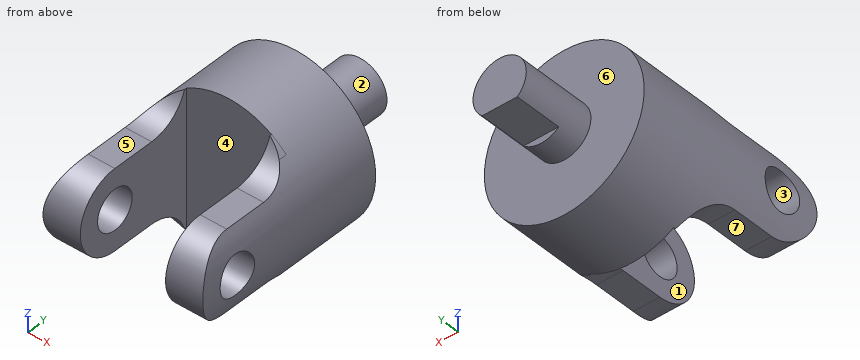
from build123d import *

# Parameters (mm, degrees)
IZIM2_R                          = 19.05
Y_KSEKLIK_EKSTR_ZYON2_DEPTH      = 18.42
Y_KSEKLIK_EKSTR_ZYON4_REACH      = 41.439
Y_KSEKLIK_EKSTR_ZYON4_END_RADIUS = 19.05
IZIM3_R                          = 4.765
RADYUS1_R                        = 9.53
IZIM5_R                          = 6.35
Y_KSEKLIK_EKSTR_ZYON5_DEPTH      = 17.81
IZIM6_W                          = 1.59
IZIM6_H                          = 11.43
KES_EKSTR_ZYON2_DEPTH            = 8.905


with BuildPart() as part:
    # Çizim2 → Yükseklik-Ekstrüzyon2 (new body)
    with BuildSketch(Plane(origin=(0, 0, 0), x_dir=(1, 0, 0), z_dir=(0, 1, 0))):
        with Locations(Location((0, 0, 0), (0, 0, 270))):
            Circle(IZIM2_R)
    extrude(amount=-Y_KSEKLIK_EKSTR_ZYON2_DEPTH)

    # Yükseklik-Ekstrüzyon4: up to this cylinder (the profile starts inside it)
    y_kseklik_ekstr_zyon4_end = Plane(origin=(0, -31.124737, 0), z_dir=(0, 1, 0)) * Cylinder(Y_KSEKLIK_EKSTR_ZYON4_END_RADIUS, 121.978, mode=Mode.PRIVATE)
    # Çizim3 → Yükseklik-Ekstrüzyon4 (add, up to the surface)
    with BuildSketch(Plane(origin=(10.16, 0, 0), x_dir=(0, 0, -1), z_dir=(1, 0, 0)), mode=Mode.PRIVATE) as y_kseklik_ekstr_zyon4_sk1:
        with BuildLine():
            Line((-9.53, -38.1), (-9.53, -18.42))
            Line((-9.53, -18.42), (9.53, -18.42))
            Line((9.53, -18.42), (9.53, -38.1))
            ThreePointArc((9.53, -38.1), (0, -47.63), (-9.53, -38.1))
        make_face()
        with Locations(Location((0, -38.1, 0), (0, 0, 180))):
            Circle(IZIM3_R, mode=Mode.SUBTRACT)
    y_kseklik_ekstr_zyon4_tool1 = extrude(y_kseklik_ekstr_zyon4_sk1.sketch, amount=Y_KSEKLIK_EKSTR_ZYON4_REACH, mode=Mode.PRIVATE) & y_kseklik_ekstr_zyon4_end
    y_kseklik_ekstr_zyon4 = y_kseklik_ekstr_zyon4_tool1.solids().sort_by_distance((10.16, -31.124737, 0))[0]
    add(y_kseklik_ekstr_zyon4)

    # Aynalama3: Yükseklik-Ekstrüzyon4 across plane
    add(y_kseklik_ekstr_zyon4.mirror(Plane(origin=(0, 0, 0), x_dir=(0, 0, 1), z_dir=(1, 0, 0))))

    # Radyus1
    # the kernel refuses this fillet: 9.53 mm, written as the material it adds along each edge
    with BuildSketch(Plane(origin=(13.665, -18.42, 9.53), x_dir=(0, 0, 1), z_dir=(-1, 0, 0))) as radyus1_piece_1_section:
        with BuildLine():
            CenterArc((RADYUS1_R, -RADYUS1_R), RADYUS1_R, 90, 90)
            Line((0, -RADYUS1_R), (0, 0))
            Line((0, 0), (RADYUS1_R, 0))
        make_face()
    radyus1_piece_1 = extrude(amount=53.98489618, mode=Mode.PRIVATE)
    radyus1_piece_1 = radyus1_piece_1 & Plane(origin=(0, -20.798311962, 0), x_dir=(0, 0, 1), z_dir=(0, 1, 0)) * Cylinder(19.05, 147, mode=Mode.PRIVATE)
    radyus1_piece_1 = split(radyus1_piece_1, bisect_by=Plane(origin=(10.16, -20.798311962, 11.199892809), z_dir=(1, 0, 0)), keep=Keep.TOP, mode=Mode.PRIVATE)
    add(radyus1_piece_1)
    with BuildSketch(Plane(origin=(-10.16, -18.42, 9.53), x_dir=(0, 0, 1), z_dir=(-1, 0, 0))) as radyus1_piece_2_section:
        with BuildLine():
            CenterArc((RADYUS1_R, -RADYUS1_R), RADYUS1_R, 90, 90)
            Line((0, -RADYUS1_R), (0, 0))
            Line((0, 0), (RADYUS1_R, 0))
        make_face()
    radyus1_piece_2 = extrude(amount=30.15989618, mode=Mode.PRIVATE)
    radyus1_piece_2 = radyus1_piece_2 & Plane(origin=(0, -21.011864307, 0), x_dir=(0, 0, 1), z_dir=(0, 1, 0)) * Cylinder(19.05, 99, mode=Mode.PRIVATE)
    add(radyus1_piece_2)
    with BuildSketch(Plane(origin=(13.665, -18.42, -9.53), x_dir=(0, 0, -1), z_dir=(-1, 0, 0))) as radyus1_piece_3_section:
        with BuildLine():
            CenterArc((RADYUS1_R, RADYUS1_R), RADYUS1_R, 180, 90)
            Line((0, RADYUS1_R), (0, 0))
            Line((0, 0), (RADYUS1_R, 0))
        make_face()
    radyus1_piece_3 = extrude(amount=53.98489618, mode=Mode.PRIVATE)
    radyus1_piece_3 = radyus1_piece_3 & Plane(origin=(0, -20.798311941, 0), x_dir=(0, 0, 1), z_dir=(0, 1, 0)) * Cylinder(19.05, 147, mode=Mode.PRIVATE)
    radyus1_piece_3 = split(radyus1_piece_3, bisect_by=Plane(origin=(10.16, -20.798311941, -11.199892873), z_dir=(1, 0, 0)), keep=Keep.TOP, mode=Mode.PRIVATE)
    add(radyus1_piece_3)
    with BuildSketch(Plane(origin=(-10.16, -18.42, -9.53), x_dir=(0, 0, -1), z_dir=(-1, 0, 0))) as radyus1_piece_4_section:
        with BuildLine():
            CenterArc((RADYUS1_R, RADYUS1_R), RADYUS1_R, 180, 90)
            Line((0, RADYUS1_R), (0, 0))
            Line((0, 0), (RADYUS1_R, 0))
        make_face()
    radyus1_piece_4 = extrude(amount=30.15989618, mode=Mode.PRIVATE)
    radyus1_piece_4 = radyus1_piece_4 & Plane(origin=(0, -21.011867626, 0), x_dir=(0, 0, 1), z_dir=(0, 1, 0)) * Cylinder(19.05, 99, mode=Mode.PRIVATE)
    add(radyus1_piece_4)
    with BuildSketch(Plane(origin=(-13.665, -18.42, 9.53), x_dir=(0, 0, 1), z_dir=(1, 0, 0))) as radyus1_piece_5_section:
        with BuildLine():
            CenterArc((RADYUS1_R, RADYUS1_R), RADYUS1_R, 180, 90)
            Line((0, RADYUS1_R), (0, 0))
            Line((0, 0), (RADYUS1_R, 0))
        make_face()
    radyus1_piece_5 = extrude(amount=53.98489618, mode=Mode.PRIVATE)
    radyus1_piece_5 = radyus1_piece_5 & Plane(origin=(0, -20.798312003, 0), x_dir=(0, 0, 1), z_dir=(0, 1, 0)) * Cylinder(19.05, 147, mode=Mode.PRIVATE)
    radyus1_piece_5 = split(radyus1_piece_5, bisect_by=Plane(origin=(-10.16, -20.798312003, 11.199892685), z_dir=(-1, 0, 0)), keep=Keep.TOP, mode=Mode.PRIVATE)
    add(radyus1_piece_5)
    with BuildSketch(Plane(origin=(10.16, -18.42, 9.53), x_dir=(0, 0, 1), z_dir=(1, 0, 0))) as radyus1_piece_6_section:
        with BuildLine():
            CenterArc((RADYUS1_R, RADYUS1_R), RADYUS1_R, 180, 90)
            Line((0, RADYUS1_R), (0, 0))
            Line((0, 0), (RADYUS1_R, 0))
        make_face()
    radyus1_piece_6 = extrude(amount=30.15989618, mode=Mode.PRIVATE)
    radyus1_piece_6 = radyus1_piece_6 & Plane(origin=(0, -21.011867621, 0), x_dir=(0, 0, 1), z_dir=(0, 1, 0)) * Cylinder(19.05, 99, mode=Mode.PRIVATE)
    add(radyus1_piece_6)
    with BuildSketch(Plane(origin=(-13.665, -18.42, -9.53), x_dir=(0, 0, -1), z_dir=(1, 0, 0))) as radyus1_piece_7_section:
        with BuildLine():
            CenterArc((RADYUS1_R, -RADYUS1_R), RADYUS1_R, 90, 90)
            Line((0, -RADYUS1_R), (0, 0))
            Line((0, 0), (RADYUS1_R, 0))
        make_face()
    radyus1_piece_7 = extrude(amount=53.98489618, mode=Mode.PRIVATE)
    radyus1_piece_7 = radyus1_piece_7 & Plane(origin=(0, -20.798311958, 0), x_dir=(0, 0, 1), z_dir=(0, 1, 0)) * Cylinder(19.05, 147, mode=Mode.PRIVATE)
    radyus1_piece_7 = split(radyus1_piece_7, bisect_by=Plane(origin=(-10.16, -20.798311958, -11.199892821), z_dir=(-1, 0, 0)), keep=Keep.TOP, mode=Mode.PRIVATE)
    add(radyus1_piece_7)
    with BuildSketch(Plane(origin=(10.16, -18.42, -9.53), x_dir=(0, 0, -1), z_dir=(1, 0, 0))) as radyus1_piece_8_section:
        with BuildLine():
            CenterArc((RADYUS1_R, -RADYUS1_R), RADYUS1_R, 90, 90)
            Line((0, -RADYUS1_R), (0, 0))
            Line((0, 0), (RADYUS1_R, 0))
        make_face()
    radyus1_piece_8 = extrude(amount=30.15989618, mode=Mode.PRIVATE)
    radyus1_piece_8 = radyus1_piece_8 & Plane(origin=(0, -21.011864338, 0), x_dir=(0, 0, 1), z_dir=(0, 1, 0)) * Cylinder(19.05, 99, mode=Mode.PRIVATE)
    add(radyus1_piece_8)

    # Çizim5 → Yükseklik-Ekstrüzyon5 (add)
    with BuildSketch(Plane(origin=(0, 0, 0), x_dir=(1, 0, 0), z_dir=(0, 1, 0))):
        with Locations(Location((0, 0, 0), (0, 0, 90))):
            Circle(IZIM5_R)
    extrude(amount=Y_KSEKLIK_EKSTR_ZYON5_DEPTH)

    # Çizim6 → Kes-Ekstrüzyon2 (cut, symmetric)
    with BuildSketch(Plane(origin=(0, 0, 0), x_dir=(0, 0, -1), z_dir=(1, 0, 0))):
        with Locations((5.555, 12.095)):
            Rectangle(IZIM6_W, IZIM6_H)
    extrude(amount=KES_EKSTR_ZYON2_DEPTH, both=True, mode=Mode.SUBTRACT)


solid = part.part
Input: part model. Units: mm. Frame: model coordinates. Face numbers are marked on the shaded views. A direction names the side the tool comes from. Coordinates: 2 decimals unless noted, no trailing zeros. Loops run counter-clockwise (first coordinate to the right, second up) from the corner with the lowest first, then second, coordinate; pieces in that order, holes last. Notation, with made-up numbers: (64, 2.25) - (82, 2.25) arc R22 cw to (82, 18.25) - close; hole circle Ø11 at (86.25, 74.5). An arc over 180 degrees is marked (long way). Answer in a Markdown table with one row per item. Add a question column.
Item 1: Section query B-B on x = 0. Return the cut outline in (y, z), then the cut area to 3 significant figures.
Item 2: Section query A-A on z = 0. Return the cut outline in (x, y) (3 decimals).
Item 3: Mould query, pull axis X, two halves, no side actions, for the marked faces 1, 2 and 3. Classes: released by +X, released by -X, zero draft, split by the parting line, or undercut.
Item 4: Line query: line 1 along Z through (x, y) = (-15.75, -38.1) (3 decimals); line 2 along Y through (x, z) = (14, 0) (3 decimals); line 3 along Y through (x, z) = (1, 16). Output: solid intervals per line, ascending. Write a range as [from, to].
Item 5: Access query for the marked faces 4, 5, 6 and 7. Directions: +Z, -Z, +X, -X, +Y, -Y. A direction counts if a zero-diameter tool reaches every point of the face in a straight line with its end or side. Return the directions, or none.
Item 6: Section query C-C on y = 2.5. Return the cut outline in (x, z).
Item 7: Contact query for flat-ended pins moving along their axis: P1, Ø4, axis at x = -1, z = 2.5, coming from the -Y side; P2, Ø1.5, axis at y = -34.5, z = 5.5, coming from the +X side; P3, Ø9, axis at y = -28.5, z = -2, coming from the +X side; P4, Ø12, axis at y = 4.5, z = -14.5, coming from the -X side. Output: stop coordinate, or through.
Item 8: Section query D-D on z = 10.5. Return the cut outline in (x, y), then the cut area to 3 significant figures.
Recorded:
| question | item | result |
|---|---|---|
| 1 | outline | (-18.42, -19.05) - (0, -19.05) - (0, -6.35) - (6.38, -6.35) - (6.38, -4.76) - (17.81, -4.76) - (17.81, 6.35) - (0, 6.35) - (0, 19.05) - (-18.42, 19.05) - close |
| 1 | area | 910 mm^2 |
| 2 | outline | (-19.05, -47.63) - (-10.16, -47.63) - (-10.16, -42.865) - (-19.05, -42.865) - close; (-19.05, -33.335) - (-10.16, -33.335) - (-10.16, -18.42) - (10.16, -18.42) - (10.16, -33.335) - (19.05, -33.335) - (19.05, 0) - (6.35, 0) - (6.35, 17.81) - (-6.35, 17.81) - (-6.35, 0) - (-19.05, 0) - close; (10.16, -47.63) - (19.05, -47.63) - (19.05, -42.865) - (10.16, -42.865) - close |
| 3 | face 1 | undercut |
| 3 | face 2 | split by the parting line |
| 3 | face 3 | zero draft |
| 4 | line 1 | [-9.53, -4.765], [4.765, 9.53] |
| 4 | line 2 | [-47.63, -42.865], [-33.335, 0] |
| 4 | line 3 | [-18.42, 0] |
| 5 | face 4 | +Z, -Z, -Y |
| 5 | face 5 | +Z, +X, -X, -Y |
| 5 | face 6 | +Y |
| 5 | face 7 | -Z, +X, -X, -Y |
| 6 | outline | circle Ø12.7 at (0, 0) |
| 7 | P1 | y = -18.42 |
| 7 | P2 | x = 18.45 |
| 7 | P3 | x = 19.05 |
| 7 | P4 | x = -15.87 |
| 8 | outline | (-15.9, -23.76) - (-10.16, -23.76) - (-10.16, -18.42) - (10.16, -18.42) - (10.16, -23.76) - (15.9, -23.76) - (15.9, 0) - (-15.9, 0) - close |
| 8 | area | 647 mm^2 |
